Geometry check sheet. Reference: drawing and pictorial views, mm from the part's lowest x, y, z. A direction names the side the tool comes from. Give positions to 0.01 mm unless a question says otherwise; leave off trailing zeros. Loops run counter-clockwise (first coordinate to the right, second up) from the corner with the lowest first, then second, coordinate; pieces in that order, holes last. Notation, with made-up numbers: (-21.5, -20) -> (25.5, -20) arc R26 ccw to (25.5, 2) -> close; hole circle Ø5 at (33, -40). An arc over 180 degrees is marked (long way). One line per item, written item: value. Start each with the question number.
(1) Sectioned sample at D-D, the plane y = 11. Record the cut outline in (x, z), then the cut area to 3 significant figures.
(2) Draft check along X on the marked faces 3, 4 and 5. Enter one of: pulls with the +X half, pulls with the -X half, needs draft (parallel to the pull), parting line crosses it, or undercut.
(3) Sectioned sample at A-A, the plane x = 6. Record the cut outline in (y, z), then the cut area to 3 significant figures.
(4) Gauge pin test, flat ends, axial feed: pin 1 Ø1.5 at (x, z) = (7, 4) entering from -Y; pin 2 Ø1.5 at (y, z) = (9, 2) entering from +X; pin 3 Ø1.5 at (x, z) = (5, 4.5) entering from +Y. Record the tip position at first contact, or that the pin passes through.
(5) Scan lines: line 1 along Y through (x, z) = (6, 2.25); line 2 along Z through (x, y) = (2.75, 1.75); line 3 along X through (y, z) = (6.5, 2). Record each from-to range of solid material in increasing order. Write a range as from..to.
(6) Tool access check on the marked faces 1 and 2. Record the directions out of +Z, -Z, +X, -X, +Y, -Y that give a thin tool (end or side, any length) a straight path to the whole face; none if there is none.
(7) Sectioned sample at C-C, the plane z = 2.25. Record the cut outline in (x, y).
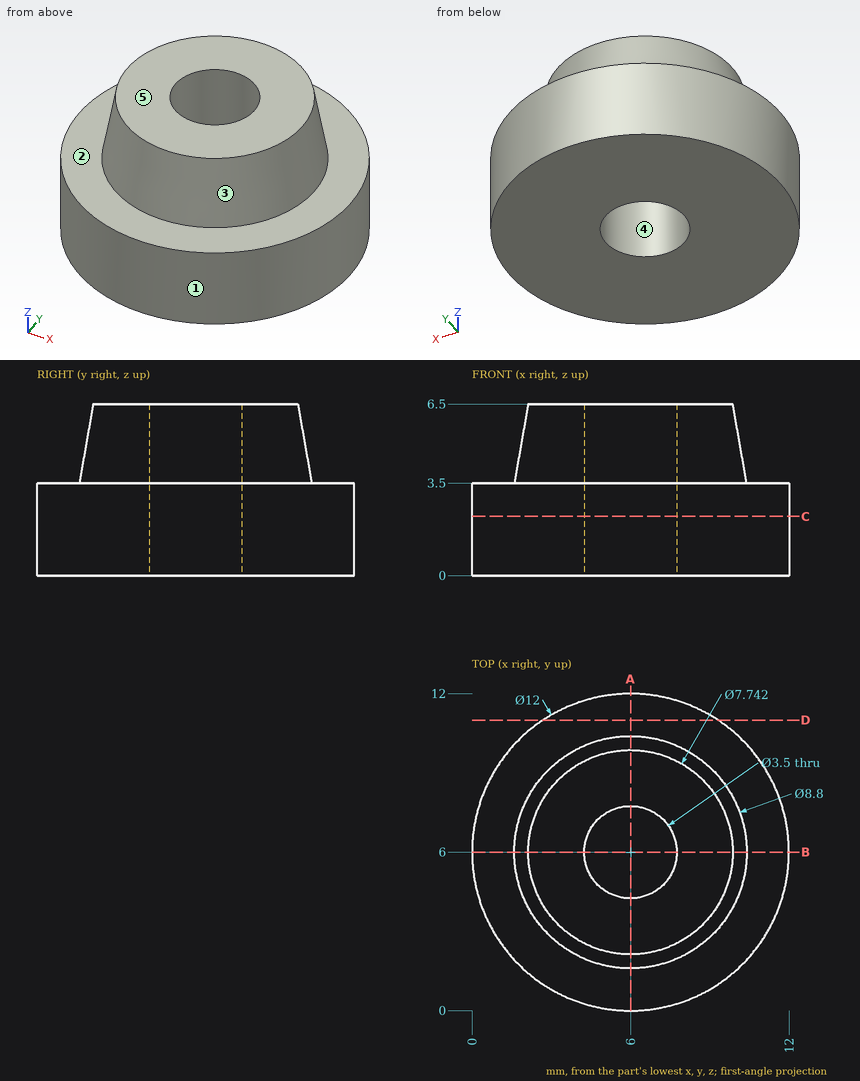
Calculated:
1. outline: (2.68, 0) -> (9.32, 0) -> (9.32, 3.5) -> (2.68, 3.5) -> close
1. area: 23.2 mm2
2. face 3: parting line crosses it
2. face 4: undercut
2. face 5: needs draft
3. outline: (0, 0) -> (4.25, 0) -> (4.25, 6.5) -> (2.13, 6.5) -> (1.6, 3.5) -> (0, 3.5) -> close; (7.75, 0) -> (12, 0) -> (12, 3.5) -> (10.4, 3.5) -> (9.87, 6.5) -> (7.75, 6.5) -> close
3. area: 44.1 mm2
4. pin 1: stops at y = 0.02
4. pin 2: stops at x = 11.56
4. pin 3: stops at y = 10.29
5. line 1: y = 0..4.25, 7.75..12
5. line 2: z = 0..3.5
5. line 3: x = 0.02..4.32, 7.68..11.98
6. face 1: +Z, -Z
6. face 2: +Z
7. outline: circle Ø12 at (6, 6); hole circle Ø3.5 at (6, 6)
